from build123d import *

# Parameters (mm, degrees)
SKETCH2_W           = 37
SKETCH2_H           = 15
BOSS_EXTRUDE1_DEPTH = 12
SKETCH3_R           = 17.5
BOSS_EXTRUDE2_DEPTH = 15
FILLET1_SIZE        = 5.5


with BuildPart() as part:
    # Sketch2 → Boss-Extrude1 (new body)
    with BuildSketch(Plane.XY):
        with Locations((-165.97258371, 72.296511628)):
            Rectangle(SKETCH2_W, SKETCH2_H)
    extrude(amount=BOSS_EXTRUDE1_DEPTH)

    # Sketch3 → Boss-Extrude2 (add)
    with BuildSketch(Plane(origin=(-147.47258371, 0, 0), x_dir=(0, 0, -1), z_dir=(1, 0, 0))):
        with Locations((-6, 72.296511628)):
            Circle(SKETCH3_R)
    extrude(amount=BOSS_EXTRUDE2_DEPTH)

    # Fillet1
    # a fillet whose section is not a circle: 5.5 mm, written as the material it takes off along each edge
    with BuildSketch(Plane(origin=(-147.47258371, 64.796511628, 0), x_dir=(0, 0, 1), z_dir=(-1, 0, 0)), Plane(origin=(-147.47258371, 64.796511628, 12), x_dir=(0, 1, 0), z_dir=(-1, 0, 0)), Plane(origin=(-198.22258371, 79.796511628, 0), x_dir=(0, 0, 1), z_dir=(1, 0, 0))) as fillet1_piece_1:
        with BuildLine():
            Bezier((FILLET1_SIZE, 0), (0, 0), (0, FILLET1_SIZE), weights=[1, 1.857142857, 1])
            Line((0, FILLET1_SIZE), (0, 0))
            Line((0, 0), (FILLET1_SIZE, 0))
        make_face()
    extrude(amount=50.75, mode=Mode.SUBTRACT)
    with BuildSketch(Plane(origin=(-198.22258371, 79.796511628, 12), x_dir=(0, 0, -1), z_dir=(1, 0, 0))) as fillet1_piece_2:
        with BuildLine():
            Bezier((FILLET1_SIZE, 0), (0, 0), (0, -FILLET1_SIZE), weights=[1, 1.857142857, 1])
            Line((0, -FILLET1_SIZE), (0, 0))
            Line((0, 0), (FILLET1_SIZE, 0))
        make_face()
    extrude(amount=50.75, mode=Mode.SUBTRACT)


solid = part.part
Design review of the part built by this model. Coordinates are the model's own, in mm. A direction names the side the tool comes from. Coordinates: 2 decimals unless noted, no trailing zeros. Order: outer loops, then holes, each group sorted by start corner. A loop starts at its lowest first (then second) coordinate and runs counter-clockwise, first axis right, second up.
Item 1: The part is to be moulded in two halves that separate along Z. For faces 1 (the flat face through (-166, 72, 0)), 2 (the flat face through (-184.473, 72, 6)), 3 (the flat face through (-166, 72, 12)), say which applies: pulls with the +Z half, pulls with the -Z half, needs draft (parallel to the pull), parting line crosses it, or undercut.
Item 2: Take a section at B-B, the plane z = 14.5. Write out the cut boundary in (x, y), then the cut area to 3 significant figures.
Item 3: Take a section at D-D, the plane y = 82. Write out the cut boundary in (x, z), then the cut area to 3 significant figures.
Item 4: Take a section at C-C, the plane x = -142.5. Write out the cut boundary in (y, z), then the cut area to 3 significant figures.
Item 5: For line 1 (X direction, y = 88.5, z = 8); line 2 (Y direction, x = -182, z = 5.5); line 3 (Y direction, x = -142.5, z = 2.5), list the stretches that pass through material, from the lowest coordinate up.
Item 6: For faces 4 (the flat face through (-147.473, 73, -2)), 5 (the flat face through (-132.473, 73, 6)), list the 3-axis set-ups (+Z, -Z, +X, -X, +Y, -Y) from which the entire face can be reached by the end or side of a thin tool; tool diameter is ignored.
Item 7: For pin 1 Ø1.2 at (x, y) = (-163.5, 72) entering from -Z; pin 2 Ø12 at (x, z) = (-158, 16.5) entering from -Y; pin 3 Ø2 at (x, y) = (-138.5, 83) entering from +Z; pin 4 Ø1.5 at (x, y) = (-152, 81.5) entering from +Z, all flat-tipped, find the tip position at first contact; note any pin that passes through.
Item 8: Take a section at A-A, the plane y = 71.5. Write out the cut boundary in (x, z), then the cut area to 3 significant figures.
The answers:
1. face 1: pulls with the -Z half
1. face 2: needs draft
1. face 3: pulls with the +Z half
2. outline: (-147.47, 57) - (-132.47, 57) - (-132.47, 87.59) - (-147.47, 87.59) - close
2. area: 459 mm2
3. outline: (-147.47, -8.56) - (-132.47, -8.56) - (-132.47, 20.56) - (-147.47, 20.56) - close
3. area: 437 mm2
4. outline: circle Ø35 at (72.3, 6)
4. area: 962 mm2
5. line 1: x = -147.47 to -132.47
5. line 2: y = 64.8 to 79.8
5. line 3: y = 55.15 to 89.44
6. face 4: -X
6. face 5: +Z, -Z, +X, +Y, -Y
7. pin 1: stops at z = 0
7. pin 2: stops at y = 65.37
7. pin 3: stops at z = 20.56
7. pin 4: passes through
8. outline: (-184.47, 0) - (-147.47, 0) - (-147.47, -11.48) - (-132.47, -11.48) - (-132.47, 23.48) - (-147.47, 23.48) - (-147.47, 12) - (-184.47, 12) - close
8. area: 968 mm2
